The model under review builds one solid part; all positions refer to its coordinate system, in mm. A direction names the side the tool comes from. Coordinates: 2 decimals unless noted, no trailing zeros. Write each loop counter-clockwise with the first axis right and the second up, starting at its lowest first coordinate (ties: lowest second). Pieces come first, ordered by that corner, then holes. Notation, with made-up numbers: M 40.5,33.25 L 73.5,33.25 A19 ccw 73.5,66.25 Z; hole C 73.25,63 d11. An arc over 180 degrees is marked long. Answer as a JSON object with one key per item and string values.
```python
from build123d import *

# Parameters (mm, degrees)
F0_R            = 5.5
F1_DEPTH        = 11
F1_TAPER        = -46
F2_R            = 16.8908334517
F3_DEPTH        = 17
F4_R            = 11
F5_DEPTH        = 22
F6_R            = 11
F7_DEPTH        = 25.4
F8_R            = 22.5
F8_R_2          = 5.5
F9_DEPTH        = 34
F11_D           = 34
F11_DEPTH       = 30
F11_TIP         = 10.2146305235
F12_D           = 20
F12_DEPTH       = 44
F12_CSINK_D     = 34
F12_CSINK_ANGLE = 46
F12_TIP         = 6.0086061903
F13_D           = 11
F13_DEPTH       = 65
F13_START       = 46.7038728
F13_TIP         = 3.3047334047


with BuildPart() as f1:
    # F0 (on Front) → F1 (new body)
    with BuildSketch(Plane.XZ):
        Circle(F0_R)
    extrude(amount=F1_DEPTH, taper=F1_TAPER)

    # F2 (on face) → F3 (join)
    with BuildSketch(Plane.XZ.offset(11)):
        Circle(F2_R)
    extrude(amount=F3_DEPTH)

    # F4 (on face) → F5 (join)
    with BuildSketch(Plane.XZ.offset(28)):
        Circle(F4_R)
    extrude(amount=F5_DEPTH)

    # F6 (on face) → F7 (join)
    with BuildSketch(Plane.XZ.offset(50)):
        Polygon((17.5, -30.3108891325), (35, 0), (17.5, 30.3108891325), (-17.5, 30.3108891325), (-35, 0), (-17.5, -30.3108891325), align=None)
        Circle(F6_R, mode=Mode.SUBTRACT)
        Circle(F6_R)
    extrude(amount=F7_DEPTH)

    # F8 (on face) → F9 (join)
    with BuildSketch(Plane.XZ.offset(75.4)):
        Circle(F8_R)
        Circle(F8_R_2, mode=Mode.SUBTRACT)
        Circle(F8_R_2)
    extrude(amount=F9_DEPTH)

    # F11
    with Locations(Plane.XZ.offset(109.4)):
        with Locations((0, 0)):
            Hole(F11_D / 2, depth=F11_DEPTH)
            with Locations((0, 0, -(F11_DEPTH + F11_TIP / 2))):  # 118° drill point
                Cone(0, F11_D / 2, F11_TIP, mode=Mode.SUBTRACT)

    # F12
    with Locations(Plane.XZ.offset(109.4)):
        with Locations((0, 0)):
            CounterSinkHole(F12_D / 2, F12_CSINK_D / 2, depth=F12_DEPTH, counter_sink_angle=F12_CSINK_ANGLE)
            with Locations((0, 0, -(F12_DEPTH + F12_TIP / 2))):  # 118° drill point
                Cone(0, F12_D / 2, F12_TIP, mode=Mode.SUBTRACT)

    # F13
    # its depths count from where the whole tool has entered the part; down to there all is cleared
    with Locations(Plane.XZ.offset(109.4).offset(-F13_START)):
        with Locations((0, 0)):
            Hole(F13_D / 2, depth=F13_DEPTH)
            with Locations((0, 0, -(F13_DEPTH + F13_TIP / 2))):  # 118° drill point
                Cone(0, F13_D / 2, F13_TIP, mode=Mode.SUBTRACT)


solid = f1.part
```
(1) Draft analysis for pull direction Z (two halves, no side actions). For faces 4 (the face through (0, -63, -30.311)), 5 (the face through (-2.199, -19.381, 16.747)), 6 (the face through (-2.263, -75.457, -10.19)), state which applies: released by +Z, released by -Z, zero draft, split by the parting line, or undercut.
Results list:
{"face 4": "released by -Z", "face 5": "split by the parting line", "face 6": "undercut"}
(2) Add section B-B on y = -73. Give the boundary of the cut face in (x, z), and give its area (3 significant figures).
Results list:
{"outline": "M -35,0 L -17.5,-30.31 L 17.5,-30.31 L 35,0 L 17.5,30.31 L -17.5,30.31 Z; hole C 0,0 d20", "area": "2,870 mm²"}
(3) Add section D-D on x = 25.5. Give the boundary of the cut face in (y, z).
Results list:
{"outline": "M -75.4,-16.45 L -50,-16.45 L -50,16.45 L -75.4,16.45 Z"}
(4) Add section C-C on y = -29.5. Give the boundary of the cut face in (x, z).
Results list:
{"outline": "C 0,0 d22; hole C 0,0 d11"}
(5) Add section A-A on x = 0. Give the boundary of the cut face in (y, z), and give its area (3 significant figures).
Results list:
{"outline": "M -109.4,-22.5 L -75.4,-22.5 L -75.4,-30.31 L -50,-30.31 L -50,-11 L -28,-11 L -28,-16.89 L -11,-16.89 L 0,-5.5 L -62.7,-5.5 L -65.4,-10 L -75.19,-10 L -79.4,-17 L -109.4,-17 Z; M -109.4,17 L -79.4,17 L -75.19,10 L -65.4,10 L -62.7,5.5 L 0,5.5 L -11,16.89 L -28,16.89 L -28,11 L -50,11 L -50,30.31 L -75.4,30.31 L -75.4,22.5 L -109.4,22.5 Z", "area": "2,310 mm²"}
(6) For faces 1 (the face through (2.17, -70.23, -9.76)), 2 (the face through (3, -109.4, 17)), 3 (the face through (15, -50, 0)), list the 3-axis set-ups (+Z, -Z, +X, -X, +Y, -Y) from which the entire face can be reached by the end or side of a thin tool; tool diameter is ignored.
Results list:
{"face 1": "-Y", "face 2": "+Z, -Z, +X, -X, -Y", "face 3": "none"}
(7) For pin 1 Ø2 at (x, z) = (20.5, -22) entering from -Y; pin 2 Ø8 at (x, z) = (-19, 14.5) entering from +Y; pin 3 Ø5 at (x, y) = (23.5, -73.5) entering from -Z, all flat-tipped, find the tip position at first contact; note any pin that passes through.
Results list:
{"pin 1": "y = -75.4", "pin 2": "y = -50", "pin 3": "z = -24.25"}
(8) Wall thickness on line 1 along Z through (x, y) = (0, -71.5); line 2 along Z through (x, y) = (0, -21); line 3 along Y through (x, z) = (-9, -14): over which ranges is each line inside the solid? List them lowest first. Write a range as from..to.
Results list:
{"line 1": "-30.31..-10, 10..30.31", "line 2": "-16.89..-5.5, 5.5..16.89", "line 3": "-79.19..-50, -28..-10.76"}
